Answer from the drawing. Dimensions are ordinates in mm from the lowest x, y and z of the part. A direction names the side the tool comes from. Give positions to 0.01 mm unless a question says otherwise; leave off trailing zeros. Write each loop counter-clockwise with the first axis right and the second up, starting at its lowest first coordinate (ties: lowest second). Pieces come first, ordered by that corner, then holes. Notation, with made-up numbers: M 71,85.5 L 78,85.5 A25 ccw 78,122.5 Z; hole C 1.25,3 d3. An arc over 180 degrees is marked long. Write each question's results on one line, items separated by ' | '. Start each with the question number.
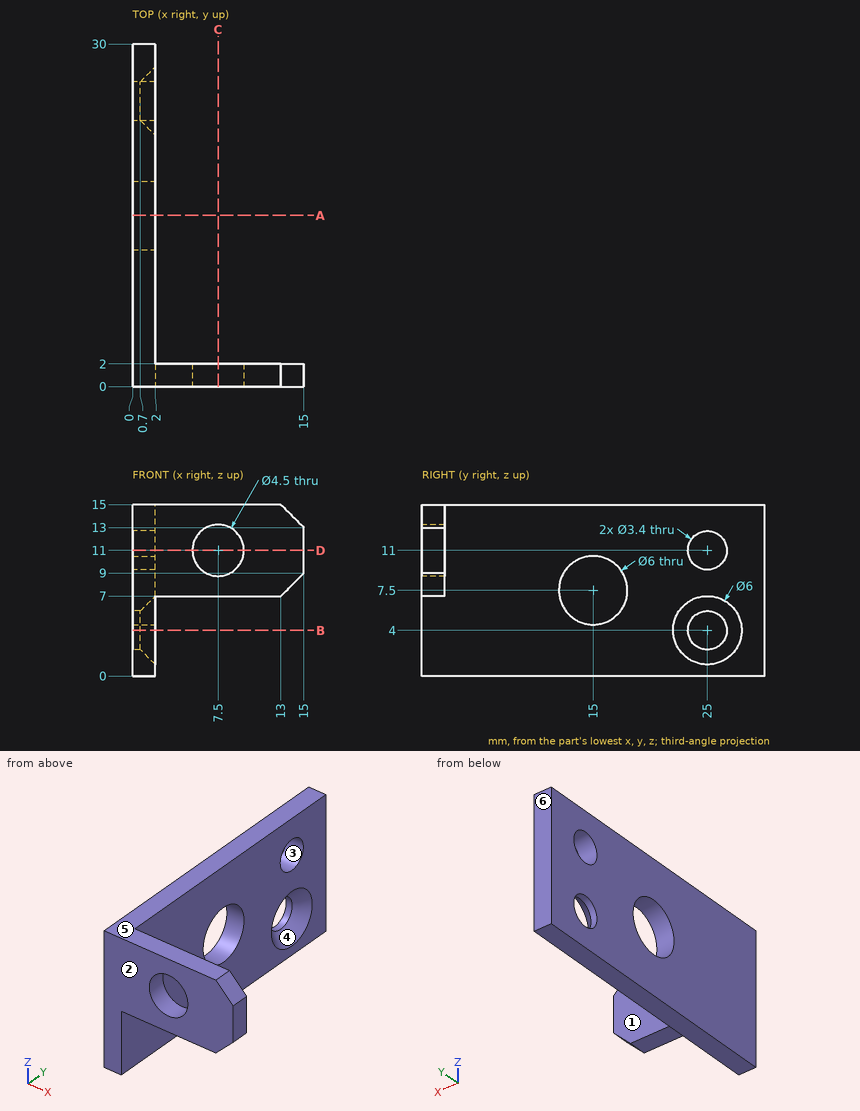
Item 1: For the marked faces 1 and 2, determine the directions among +Z, -Z, +X, -X, +Y, -Y from which every point of the face is accessible in a straight line to the end or side of a thin tool.
Item 2: Straight lines are drawn through the part: line 1 (Z direction, x = 7.5, y = 1.15); line 2 (Z direction, x = 0.5, y = 15); line 3 (Z direction, x = 0.9, y = 25). For each, find the intervals that lie inside material, in ascending order.
Item 3: Section B-B, the plane z = 4 is taken. Determine the outline of the cut face in (x, y), then the cut area to 3 significant figures.
Item 4: Given P1, Ø3, axis at y = 12, z = 6.5, coming from the +X side; P2, Ø4, axis at x = 7.5, z = 10, coming from the -Y side; P3, Ø4, axis at x = 9, z = 11, coming from the +Y side; P4, Ø0.6, axis at x = 5, y = 0.5, coming from the -Z side, each flat-ended and moving along its own axis, determine where each tip first touches the part or whether it passes through.
Item 5: Section A-A, the plane y = 15 is taken. Determine the outline of the cut face in (x, z).
Item 6: Section C-C, the plane x = 7.5 is taken. Determine the outline of the cut face in (y, z).
Item 7: Section D-D, the plane z = 11 is taken. Determine the outline of the cut face in (x, y).
Item 8: Determine the mould class of the marked faces 3, 4, 5 and 6 for opening direction Y: +Y half, -Y half, draft (parallel to the pull), parting line (faces both ways), or undercut.
Worked out:
1) face 1: +Z, -Z, +X, +Y | face 2: +Z, -Z, +X, -X, -Y
2) line 1: z = 7 to 8.75, 13.25 to 15 | line 2: z = 0 to 4.5, 10.5 to 15 | line 3: z = 0 to 2.1, 5.9 to 9.3, 12.7 to 15
3) outline: M 0,0 L 2,0 L 2,22 L 0.7,23.3 L 0,23.3 Z; M 0,26.7 L 0.7,26.7 L 2,28 L 2,30 L 0,30 Z | area: 51.5 mm²
4) P1: stops at x = 2 | P2: stops at y = 0 | P3: stops at y = 2 | P4: stops at z = 7
5) outline: M 0,0 L 2,0 L 2,4.5 L 0,4.5 Z; M 0,10.5 L 2,10.5 L 2,15 L 0,15 Z
6) outline: M 0,7 L 2,7 L 2,8.75 L 0,8.75 Z; M 0,13.25 L 2,13.25 L 2,15 L 0,15 Z
7) outline: M 0,0 L 5.25,0 L 5.25,2 L 2,2 L 2,23.3 L 0,23.3 Z; M 0,26.7 L 2,26.7 L 2,30 L 0,30 Z; M 9.75,0 L 15,0 L 15,2 L 9.75,2 Z
8) face 3: undercut | face 4: undercut | face 5: draft | face 6: +Y half
